Can you work these out from the drawing? Everything is in mm from the part's minimum corner. A direction names the side the tool comes from. Give positions to 0.01 mm unless a question says otherwise; leave off trailing zeros. Order: outer loops, then holes, each group sorted by start corner. A loop starts at its lowest first (then second) coordinate and runs counter-clockwise, first axis right, second up. Notation, with made-up numbers: (-11.75, 32) -> (41.25, 32) arc R15 ccw to (41.25, 59) -> close; hole circle Ø5 at (45.25, 58.25). An arc over 180 degrees is marked (long way). One line per item, written item: value.
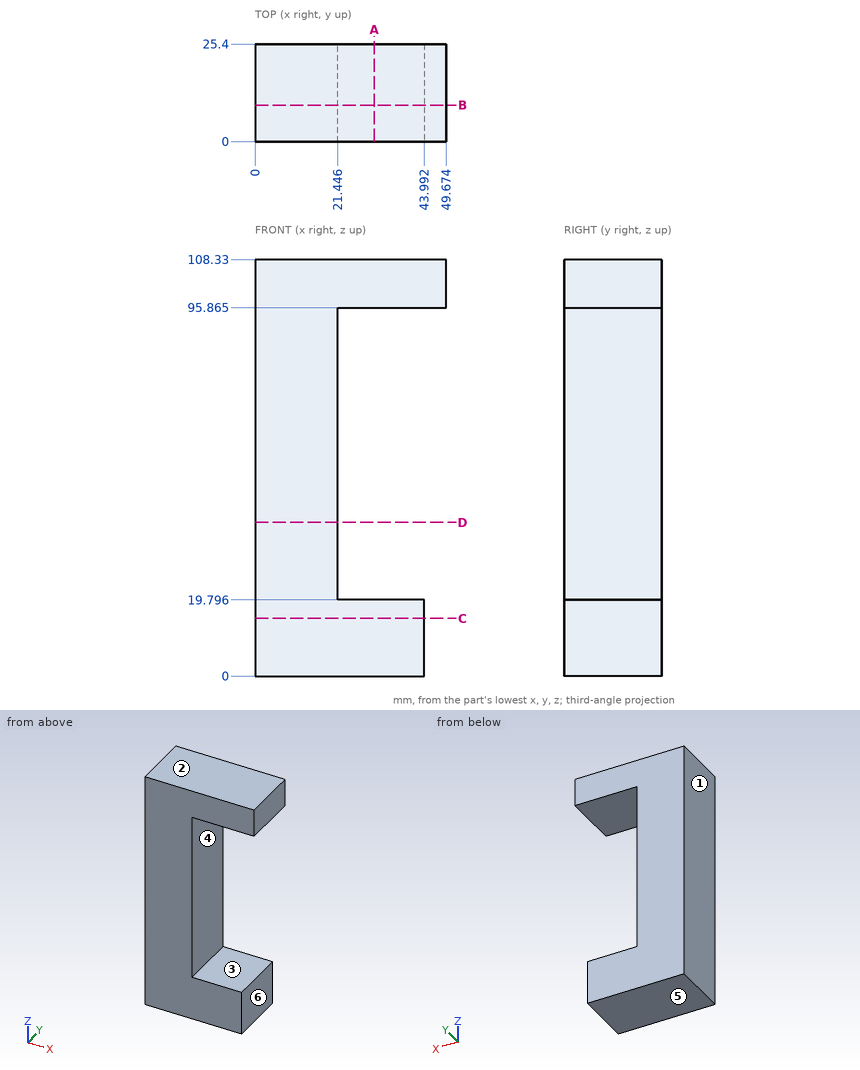
1) We'd pull the mould along Z, two halves only. Please class the marked faces 1, 2 and 3: +Z half, -Z half, draft (parallel to the pull), parting line (faces both ways), or undercut.
Answer below:
face 1: draft
face 2: +Z half
face 3: undercut
2) For the marked faces 4, 5 and 6, which set-ups out of +Z, -Z, +X, -X, +Y, -Y let a thin tool reach every point of the face, with its end or its side?
Answer below:
face 4: +X, +Y, -Y
face 5: -Z, +X, -X, +Y, -Y
face 6: -Z, +X, +Y, -Y
3) Suppose I cut it at B-B, the plane y = 9.5. Write out the boundary of the cut face in (x, z) (1 decimal).
Answer below:
outline: (0, 0) -> (44, 0) -> (44, 19.8) -> (21.4, 19.8) -> (21.4, 95.9) -> (49.7, 95.9) -> (49.7, 108.3) -> (0, 108.3) -> close
4) If I drill on line 1 along Z through (x, y) = (39, 15.25) (1 decimal); line 2 along X through (y, z) = (19.5, 51); line 3 along Z through (x, y) = (45.5, 18) (1 decimal), over which ranges is the centre line in solid material (lowest first)?
Answer below:
line 1: z = 0 to 19.8, 95.9 to 108.3
line 2: x = 0 to 21.45
line 3: z = 95.9 to 108.3
5) For P1, Ø12.5, axis at y = 12, z = 76.5, coming from the +X side, with a flat end and sliding along its axis, tell me the tip position at first contact or that it passes through.
Answer below:
P1: stops at x = 21.45
6) Suppose I cut it at A-A, the plane x = 31. Write out the boundary of the cut face in (y, z) (1 decimal).
Answer below:
outline: (0, 0) -> (25.4, 0) -> (25.4, 19.8) -> (0, 19.8) -> close; (0, 95.9) -> (25.4, 95.9) -> (25.4, 108.3) -> (0, 108.3) -> close
7) Suppose I cut it at D-D, the plane z = 40. Write out the boundary of the cut face in (x, y).
Answer below:
outline: (0, 0) -> (21.45, 0) -> (21.45, 25.4) -> (0, 25.4) -> close
8) Suppose I cut it at C-C, the plane z = 15. Write out the boundary of the cut face in (x, y), then the cut area to 3 significant figures.
Answer below:
outline: (0, 0) -> (43.99, 0) -> (43.99, 25.4) -> (0, 25.4) -> close
area: 1,120 mm2
